Here's how the part is built. I have some questions about the finished solid (model axes, mm). Face numbers are marked on the shaded views. Round coordinates to 2 decimals unless told otherwise and drop trailing zeros. Order: outer loops, then holes, each group sorted by start corner. A loop starts at its lowest first (then second) coordinate and runs counter-clockwise, first axis right, second up. Notation, with made-up numbers: (83, 44.25) - (103, 44.25) arc R31 ccw to (103, 83.25) - close; hole circle Ø5 at (21, 8). An arc over 180 degrees is marked (long way). One line per item, written item: value.
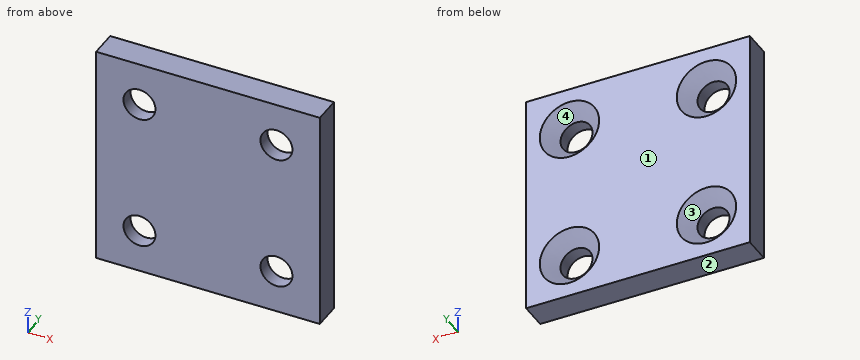
from build123d import *

# Parameters (mm, degrees)
SKETCH_1_W                  = 24.5
SKETCH_1_H                  = 24.5
SKETCH_1_R                  = 1.75
EXTRUDE_1_DEPTH             = 3
HOLE_WIZARD_M3_1_AT_2_COUNT = 2
HOLE_WIZARD_M3_1_AT_2_PITCH = 15
HOLE_WIZARD_M3_1_AT_3_COUNT = 2
HOLE_WIZARD_M3_1_AT_3_PITCH = 21.213203436
HOLE_WIZARD_M3_1_AT_4_COUNT = 2
HOLE_WIZARD_M3_1_AT_4_PITCH = 15


with BuildPart() as part:
    # 草图1 → 凸台-拉伸1 (new body)
    with BuildSketch(Plane(origin=(0, 0, 0), x_dir=(1, 0, 0), z_dir=(0, 1, 0))):
        with Locations((7.5, 7.5)):
            Rectangle(SKETCH_1_W, SKETCH_1_H)
        with Locations(Location((0, 0, 0), (0, 0, 270))):
            Circle(SKETCH_1_R, mode=Mode.SUBTRACT)
        with Locations(Location((15, 0, 0), (0, 0, 270))):
            Circle(SKETCH_1_R, mode=Mode.SUBTRACT)
        with Locations(Location((0, 15, 0), (0, 0, 270))):
            Circle(SKETCH_1_R, mode=Mode.SUBTRACT)
        with Locations(Location((15, 15, 0), (0, 0, 270))):
            Circle(SKETCH_1_R, mode=Mode.SUBTRACT)
    extrude(amount=EXTRUDE_1_DEPTH)

    # 草图5 → M3 平头机械螺钉的锥形沉头孔1 (revolve, cut)
    with BuildSketch(Plane(origin=(0, 3, 0), x_dir=(0, 0, 1), z_dir=(1, 0, 0))):
        Polygon((0, 0), (0, 3), (1.6, 3), (1.6, 1.65), (3.25, 0), align=None)
    hole_wizard_m3_1 = revolve(axis=Axis((0, 9.35, 0), (0, -1, 0)), mode=Mode.SUBTRACT)

    # M3 平头机械螺钉的锥形沉头孔1 at 2: M3 平头机械螺钉的锥形沉头孔1 ×2
    with Locations(*[(i * HOLE_WIZARD_M3_1_AT_2_PITCH, 0, 0) for i in range(1, HOLE_WIZARD_M3_1_AT_2_COUNT)]):
        add(hole_wizard_m3_1, mode=Mode.SUBTRACT)

    # M3 平头机械螺钉的锥形沉头孔1 at 3: M3 平头机械螺钉的锥形沉头孔1 ×2
    with Locations(*[Vector(0.7071067811865476, 0, -0.7071067811865476) * (i * HOLE_WIZARD_M3_1_AT_3_PITCH) for i in range(1, HOLE_WIZARD_M3_1_AT_3_COUNT)]):
        add(hole_wizard_m3_1, mode=Mode.SUBTRACT)

    # M3 平头机械螺钉的锥形沉头孔1 at 4: M3 平头机械螺钉的锥形沉头孔1 ×2
    with Locations(*[(0, 0, -i * HOLE_WIZARD_M3_1_AT_4_PITCH) for i in range(1, HOLE_WIZARD_M3_1_AT_4_COUNT)]):
        add(hole_wizard_m3_1, mode=Mode.SUBTRACT)


solid = part.part
Q1. If we section it at A-A, the plane x = 15: Please give me the cut outline in (y, z).
Results list:
outline: (0, -19.75) - (3, -19.75) - (3, -18.25) - (1.5, -16.75) - (0, -16.75) - close; (0, -13.25) - (1.5, -13.25) - (3, -11.75) - (3, -3.25) - (1.5, -1.75) - (0, -1.75) - close; (0, 1.75) - (1.5, 1.75) - (3, 3.25) - (3, 4.75) - (0, 4.75) - close
Q2. If we section it at C-C, the plane y = 2.4: Please give me the cut outline in (x, z), then the cut area to 3 significant figures.
Results list:
outline: (-4.75, -19.75) - (19.75, -19.75) - (19.75, 4.75) - (-4.75, 4.75) - close; hole circle Ø5.3 at (0, -15); hole circle Ø5.3 at (0, 0); hole circle Ø5.3 at (15, -15); hole circle Ø5.3 at (15, 0)
area: 512 mm²
Q3. If I drill on line 1 along X through (y, z) = (0.6, -15); line 2 along X through (y, z) = (1.35, -1.5); line 3 along Z through (x, y) = (17, 2.7), over which ranges is the centre line in solid material (lowest first)?
Results list:
line 1: -4.75 to -1.75, 1.75 to 13.25, 16.75 to 19.75
line 2: -4.75 to -0.9, 0.9 to 14.1, 15.9 to 19.75
line 3: -19.75 to -17.17, -12.83 to -2.17, 2.17 to 4.75
Q4. If we section it at D-D, the plane y = 0.4: Please give me the cut outline in (x, z), then the cut area to 3 significant figures.
Results list:
outline: (-4.75, -19.75) - (19.75, -19.75) - (19.75, 4.75) - (-4.75, 4.75) - close; hole circle Ø3.5 at (0, -15); hole circle Ø3.5 at (0, 0); hole circle Ø3.5 at (15, -15); hole circle Ø3.5 at (15, 0)
area: 562 mm²
Q5. We'd pull the mould along Z, two halves only. Please class the marked faces 1, 2, 3 and 4: released by +Z, released by -Z, zero draft, split by the parting line, or undercut.
Results list:
face 1: zero draft
face 2: released by -Z
face 3: undercut
face 4: undercut
Q6. If we section it at B-B, the plane z = 0: Please give me the cut outline in (x, y), then the cut area to 3 significant figures.
Results list:
outline: (-4.75, 0) - (-1.75, 0) - (-1.75, 1.5) - (-3.25, 3) - (-4.75, 3) - close; (1.75, 0) - (13.25, 0) - (13.25, 1.5) - (11.75, 3) - (3.25, 3) - (1.75, 1.5) - close; (16.75, 0) - (19.75, 0) - (19.75, 3) - (18.25, 3) - (16.75, 1.5) - close
area: 48.0 mm²
